Here's the drawing with two shaded views (mm, measured from the low corner). I have some questions. A direction names the side the tool comes from. Round coordinates to 2 decimals unless told otherwise and drop trailing zeros. Loops run counter-clockwise (first coordinate to the right, second up) from the corner with the lowest first, then second, coordinate; pieces in that order, holes last. Notation, with made-up numbers: (-14, -16.5) -> (8, -16.5) arc R27 cw to (8, 6.5) -> close; hole circle Ø2 at (65, -17.75). An arc over 180 degrees is marked (long way). Use a Markdown table: item, result.
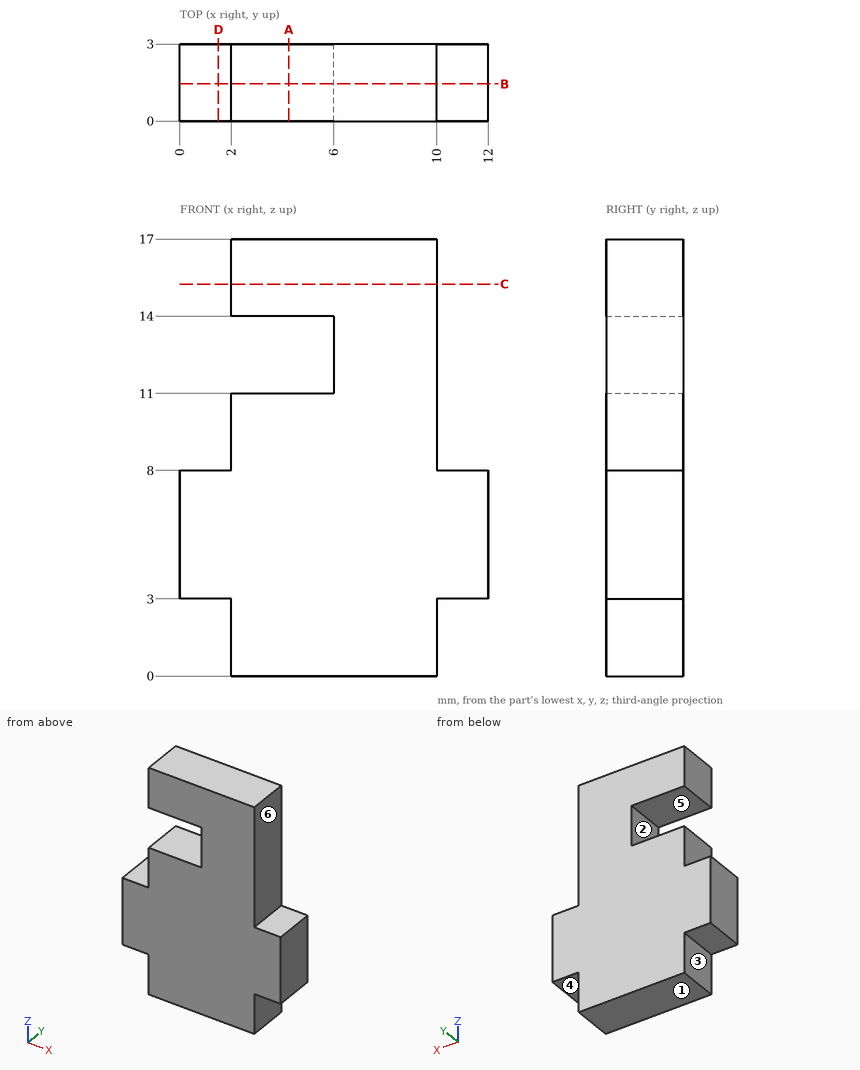
1. Will these pins go through, and if not, where does the flat tip stop? pin 1 Ø0.9 at (y, z) = (1, 2) entering from -X; pin 2 Ø0.6 at (x, y) = (0.5, 2) entering from -Z; pin 3 Ø1.5 at (y, z) = (2, 12.5) entering from -X.
Answer sheet:
| item | result |
|---|---|
| pin 1 | stops at x = 2 |
| pin 2 | stops at z = 3 |
| pin 3 | stops at x = 6 |
2. I want a section at A-A (x = 4.25). Please give me the cut outline in (y, z).
Answer sheet:
| item | result |
|---|---|
| outline | (0, 0) -> (3, 0) -> (3, 11) -> (0, 11) -> close; (0, 14) -> (3, 14) -> (3, 17) -> (0, 17) -> close |
3. I want a section at B-B (y = 1.45). Please give me the cut outline in (x, z), plus the area to 3 significant figures.
Answer sheet:
| item | result |
|---|---|
| outline | (0, 3) -> (2, 3) -> (2, 0) -> (10, 0) -> (10, 3) -> (12, 3) -> (12, 8) -> (10, 8) -> (10, 17) -> (2, 17) -> (2, 14) -> (6, 14) -> (6, 11) -> (2, 11) -> (2, 8) -> (0, 8) -> close |
| area | 144 mm² |
4. I need wall thicknesses on line 1 (Z direction, x = 5.25, y = 2.45); line 2 (Z direction, x = 11.75, y = 1.4); line 3 (X direction, y = 0.7, z = 8.5). Which ranges of each line are inside material? Lowest first, please.
Answer sheet:
| item | result |
|---|---|
| line 1 | z = 0 to 11, 14 to 17 |
| line 2 | z = 3 to 8 |
| line 3 | x = 2 to 10 |
5. Which directions (+Z, -Z, +X, -X, +Y, -Y) give clear straight access to the entire face, cutting with the end or side of a thin tool? Please do the marked faces 4, 5 and 6.
Answer sheet:
| item | result |
|---|---|
| face 4 | -Z, +X, +Y, -Y |
| face 5 | -X, +Y, -Y |
| face 6 | +Z, +X, +Y, -Y |
6. I want a section at C-C (z = 15.25). Please give me the cut outline in (x, y).
Answer sheet:
| item | result |
|---|---|
| outline | (2, 0) -> (10, 0) -> (10, 3) -> (2, 3) -> close |
7. I want a section at D-D (x = 1.5). Please give me the cut outline in (y, z).
Answer sheet:
| item | result |
|---|---|
| outline | (0, 3) -> (3, 3) -> (3, 8) -> (0, 8) -> close |
8. If we mould it in two halves opening along Z, with no side actions, what happens to the marked faces 1, 2 and 3? For each: +Z half, -Z half, draft (parallel to the pull), parting line (faces both ways), or undercut.
Answer sheet:
| item | result |
|---|---|
| face 1 | -Z half |
| face 2 | undercut |
| face 3 | draft |
